from build123d import *

# Parameters (mm, degrees)
F1_DEPTH = 127
F1_TAPER = 3
F3_DEPTH = 25.4


with BuildPart() as f1:
    # F0 (on Top) → F1 (new body, symmetric)
    with BuildSketch(Plane.XY):
        with BuildLine():
            Line((-50.8, -50.8), (50.8, -50.8))
            Line((50.8, -50.8), (50.8, 50.8))
            ThreePointArc((50.8, 50.8), (0, 101.6), (-50.8, 50.8))
            Line((-50.8, 50.8), (-50.8, -50.8))
        make_face()
    extrude(amount=F1_DEPTH, both=True, taper=F1_TAPER)

    # F2 (on face) → F3 (join)
    with BuildSketch(Plane.XY.offset(127)):
        with BuildLine():
            ThreePointArc((44.1442120311, 50.8), (0, 94.9442120311), (-44.1442120311, 50.8))
            Line((-44.1442120311, 50.8), (-44.1442120311, -44.1442120311))
            Line((-44.1442120311, -44.1442120311), (44.1442120311, -44.1442120311))
            Line((44.1442120311, -44.1442120311), (44.1442120311, 50.8))
        make_face()
        Polygon((-21.4192807622, -16.6554342237), (-21.4192807622, 8.7445657763), (0, 20.0903888761), (17.8153019142, 8.7445657763), (17.8153019142, -16.6554342237), align=None, mode=Mode.SUBTRACT)
    extrude(amount=F3_DEPTH)


solid = f1.part
Geometry: final body of the model. Coordinates: model frame, mm. A direction names the side the tool comes from. Round coordinates to 2 decimals unless told otherwise and drop trailing zeros. Write each loop counter-clockwise with the first axis right and the second up, starting at its lowest first coordinate (ties: lowest second). Pieces come first, ordered by that corner, then holes. Notation, with made-up numbers: M -25.75,63.5 L -18.75,63.5 A18 ccw -18.75,69.5 Z; hole C 80.5,10.5 d7. An arc over 180 degrees is marked long. Write item = value, one per line.
Item 1: Section query B-B on z = 22.5. Return loops of the section in (x, y).
Findings:
outline = M -49.62,-49.62 L 49.62,-49.62 L 49.62,50.8 A49.62 ccw -49.62,50.8 Z
Item 2: Pin query (flat end, axial travel): P1, Ø12.5, axis at y = -9.5, z = 135, coming from the -X side; P2, Ø7.5, axis at y = 17, z = 145.5, coming from the +X side; P3, Ø20.5, axis at x = -18.5, z = 136.5, coming from the -Y side. Return the tip coordinate at first contact, or that it passes through.
Findings:
P1 = -44.14
P2 = 44.14
P3 = -44.18
Item 3: Pull-direction query (Y, two-part tool) for faces 1 (the face through (17.815, -4, 140)), 2 (the face through (1.043, 98.214, 64.389)), 3 (the face through (47.52, 0.71, 62.61)), 4 (the face through (-21.419, -4, 140)); classes: pulls with the +Y half, pulls with the -Y half, needs draft (parallel to the pull), parting line crosses it, or undercut.
Findings:
face_1 = undercut
face_2 = pulls with the +Y half
face_3 = needs draft
face_4 = undercut
Item 4: Access query for faces 5 (the face through (-10.86, 14.34, 139.52)), 6 (the face through (0.971, 94.934, 139.522)), 7 (the face through (-44.144, 4, 140)). Directions: +Z, -Z, +X, -X, +Y, -Y. A direction counts if a zero-diameter tool reaches every point of the face in a straight line with its end or side. Return the directions, or none.
Findings:
face_5 = +Z
face_6 = +Z, +Y
face_7 = +Z, -X, +Y, -Y
Item 5: Material intervals for line 1 along Y through (x, z) = (-20.5, 60.5); line 2 along Y through (x, z) = (-7, -114.5); line 3 along X through (y, z) = (54.5, 137), sorted ascending. Write a range as [from, to].
Findings:
line_1 = [-47.63, 93.79]
line_2 = [-44.8, 95.05]
line_3 = [-43.99, 43.99]
Item 6: Section query A-A on z = 62. Return loops of the section in (x, y).
Findings:
outline = M -47.55,-47.55 L 47.55,-47.55 L 47.55,50.8 A47.55 ccw -47.55,50.8 Z
